Part model, mm, in its own coordinate system. Coordinates: 2 decimals unless noted, no trailing zeros. Loops run counter-clockwise (first coordinate to the right, second up) from the corner with the lowest first, then second, coordinate; pieces in that order, holes last. Notation, with made-up numbers: (57, 58) - (67, 58) arc R8 ccw to (67, 68) - close; hole circle Ø8 at (6, -9). An arc over 180 degrees is marked (long way). Use a Markdown table: item, result. Add a question column.
1. Band-saw the part on A-A, the plane x = 99.5. Give the cut face in (y, z).
2. Band-saw the part on B-B, the plane y = 123.19. Give the cut face in (x, z).
3. Band-saw the part on C-C, the plane y = 55. Give the cut face in (x, z), plus the area to 3 significant figures.
4. Wall check: probe 1 along Y at (x, z) = (113.5, 2.5); probe 2 along Y at (x, z) = (139, 2); probe 3 along X at (y, z) = (88.5, 1.3) (1 decimal). Give the ranges that are in metal, low to high. Write a range as [from, to].
5. Drop flat-ended pins along their axis: pin 1 (2 mm diameter, centred on x = 123.5, z = 2.5, fed in from -Y); pin 2 (2 mm diameter, centred on y = 169.5, z = 1.5, fed in from +X); pin 3 (2 mm diameter, centred on x = 245.5, z = 3, fed in from +Y). Give the stop position or say it passes through.
6. Band-saw the part on D-D, the plane z = 0.9. Count the separate pieces of the cut face and the enclosed holes in it, plus the area to 3 significant figures.
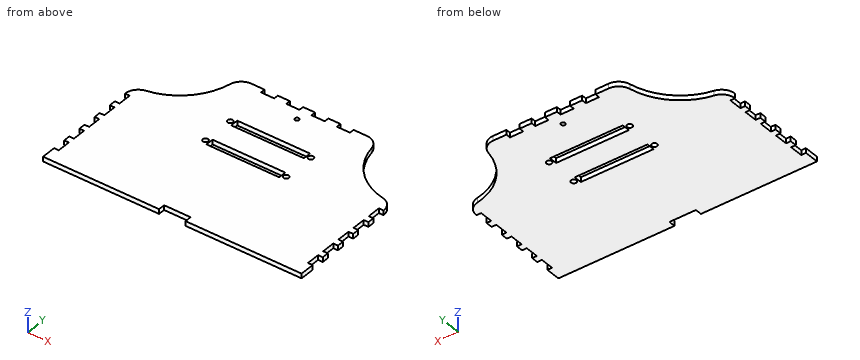
from build123d import *

# Parameters (mm, degrees)
BOSS_EXTRUDE1_DEPTH = 4.4958
FILLET1_R           = 12.7
SKETCH2_W           = 4.4958
SKETCH2_H           = 12.7
CUT_EXTRUDE1_DEPTH  = 302.762747772
SKETCH3_W           = 12.7
SKETCH3_H           = 4.4958
CUT_EXTRUDE2_DEPTH  = 302.762747772
SKETCH5_W           = 25.4
SKETCH5_H           = 6.35
CUT_EXTRUDE4_DEPTH  = 302.762747772
SKETCH7_R           = 2.54
SKETCH7_W           = 69.85
SKETCH7_H           = 7.62
CUT_EXTRUDE6_DEPTH  = 302.762747772
SKETCH8_R           = 2
CUT_EXTRUDE7_DEPTH  = 302.762747772


with BuildPart() as part:
    # Sketch1 → Boss-Extrude1 (new body)
    with BuildSketch(Plane.XY):
        with BuildLine():
            Line((0, 114.3), (0, 0))
            Line((0, 0), (248.285, 0))
            Line((248.285, 0), (248.285, 114.3))
            ThreePointArc((248.285, 114.3), (207.873847455, 131.038847455), (191.135, 171.45))
            Line((191.135, 171.45), (57.15, 171.45))
            ThreePointArc((57.15, 171.45), (40.411152545, 131.038847455), (0, 114.3))
        make_face()
    extrude(amount=BOSS_EXTRUDE1_DEPTH)

    # Fillet1
    fillet1_edges = [part.edges().sort_by_distance(p)[0] for p in [
        (248.285, 114.3, 2.2479),
        (0, 114.3, 2.2479),
        (57.15, 171.45, 2.2479),
        (191.135, 171.45, 2.2479),
    ]]
    fillet(fillet1_edges, radius=FILLET1_R)

    # Sketch2 → Cut-Extrude1 (cut, through all)
    with BuildSketch(Plane.XY.offset(4.4958)):
        with Locations((246.0371, 96.414248202)):
            Rectangle(SKETCH2_W, SKETCH2_H)
        with Locations((246.0371, 77.364248202)):
            Rectangle(SKETCH2_W, SKETCH2_H)
        with Locations((246.0371, 39.264248202)):
            Rectangle(SKETCH2_W, SKETCH2_H)
        with Locations((246.0371, 58.314248202)):
            Rectangle(SKETCH2_W, SKETCH2_H)
        with Locations((246.0371, 20.214248202)):
            Rectangle(SKETCH2_W, SKETCH2_H)
        with Locations((2.2479, 96.414248202)):
            Rectangle(SKETCH2_W, SKETCH2_H)
        with Locations((2.2479, 77.364248202)):
            Rectangle(SKETCH2_W, SKETCH2_H)
        with Locations((2.2479, 58.314248202)):
            Rectangle(SKETCH2_W, SKETCH2_H)
        with Locations((2.2479, 39.264248202)):
            Rectangle(SKETCH2_W, SKETCH2_H)
        with Locations((2.2479, 20.214248202)):
            Rectangle(SKETCH2_W, SKETCH2_H)
    extrude(amount=-CUT_EXTRUDE1_DEPTH, mode=Mode.SUBTRACT)

    # Sketch3 → Cut-Extrude2 (cut, through all)
    with BuildSketch(Plane.XY.offset(4.4958)):
        with Locations((112.006917266, 169.2021)):
            Rectangle(SKETCH3_W, SKETCH3_H)
        with Locations((87.735751798, 169.2021)):
            Rectangle(SKETCH3_W, SKETCH3_H)
        with Locations((136.278082734, 169.2021)):
            Rectangle(SKETCH3_W, SKETCH3_H)
        with Locations((160.549248202, 169.2021)):
            Rectangle(SKETCH3_W, SKETCH3_H)
    extrude(amount=-CUT_EXTRUDE2_DEPTH, mode=Mode.SUBTRACT)

    # Sketch5 → Cut-Extrude4 (cut, through all)
    with BuildSketch(Plane.XY.offset(4.4958)):
        with Locations((124.1425, 3.175)):
            Rectangle(SKETCH5_W, SKETCH5_H)
    extrude(amount=-CUT_EXTRUDE4_DEPTH, mode=Mode.SUBTRACT)

    # Sketch7 → Cut-Extrude6 (cut, through all)
    with BuildSketch(Plane(origin=(0, 0, 0), x_dir=(-1, 0, 0), z_dir=(0, 0, -1))):
        with Locations((-85.4075, 123.19)):
            Circle(SKETCH7_R)
        with Locations((-162.8775, 123.19)):
            Circle(SKETCH7_R)
        with Locations((-124.1425, 123.19)):
            Rectangle(SKETCH7_W, SKETCH7_H)
        with Locations((-124.1425, 92.202)):
            Rectangle(SKETCH7_W, SKETCH7_H)
        with Locations((-85.4075, 92.202)):
            Circle(SKETCH7_R)
        with Locations((-162.8775, 92.202)):
            Circle(SKETCH7_R)
    extrude(amount=-CUT_EXTRUDE6_DEPTH, mode=Mode.SUBTRACT)

    # Sketch8 → Cut-Extrude7 (cut, through all)
    with BuildSketch(Plane(origin=(0, 0, 0), x_dir=(-1, 0, 0), z_dir=(0, 0, -1))):
        with Locations((-124.1425, 156.21)):
            Circle(SKETCH8_R)
    extrude(amount=-CUT_EXTRUDE7_DEPTH, mode=Mode.SUBTRACT)


solid = part.part
Geometry check:
| question | item | result |
|---|---|---|
| 1 | outline | (0, 0) - (88.39, 0) - (88.39, 4.5) - (0, 4.5) - close; (96.01, 0) - (119.38, 0) - (119.38, 4.5) - (96.01, 4.5) - close; (127, 0) - (171.45, 0) - (171.45, 4.5) - (127, 4.5) - close |
| 2 | outline | (30.61, 0) - (82.87, 0) - (82.87, 4.5) - (30.61, 4.5) - close; (87.95, 0) - (89.22, 0) - (89.22, 4.5) - (87.95, 4.5) - close; (159.07, 0) - (160.34, 0) - (160.34, 4.5) - (159.07, 4.5) - close; (165.42, 0) - (217.67, 0) - (217.67, 4.5) - (165.42, 4.5) - close |
| 3 | outline | (4.5, 0) - (243.79, 0) - (243.79, 4.5) - (4.5, 4.5) - close |
| 3 | area | 1,080 mm^2 |
| 4 | probe 1 | y = [6.35, 88.39], [96.01, 119.38], [127, 166.95] |
| 4 | probe 2 | y = [0, 88.39], [96.01, 119.38], [127, 166.95] |
| 4 | probe 3 | x = [0, 89.2], [159.1, 248.3] |
| 5 | pin 1 | stops at y = 6.35 |
| 5 | pin 2 | stops at x = 187.74 |
| 5 | pin 3 | stops at y = 111.81 |
| 6 | separate pieces | 1 |
| 6 | enclosed holes | 7 |
| 6 | area | 35,200 mm^2 |
